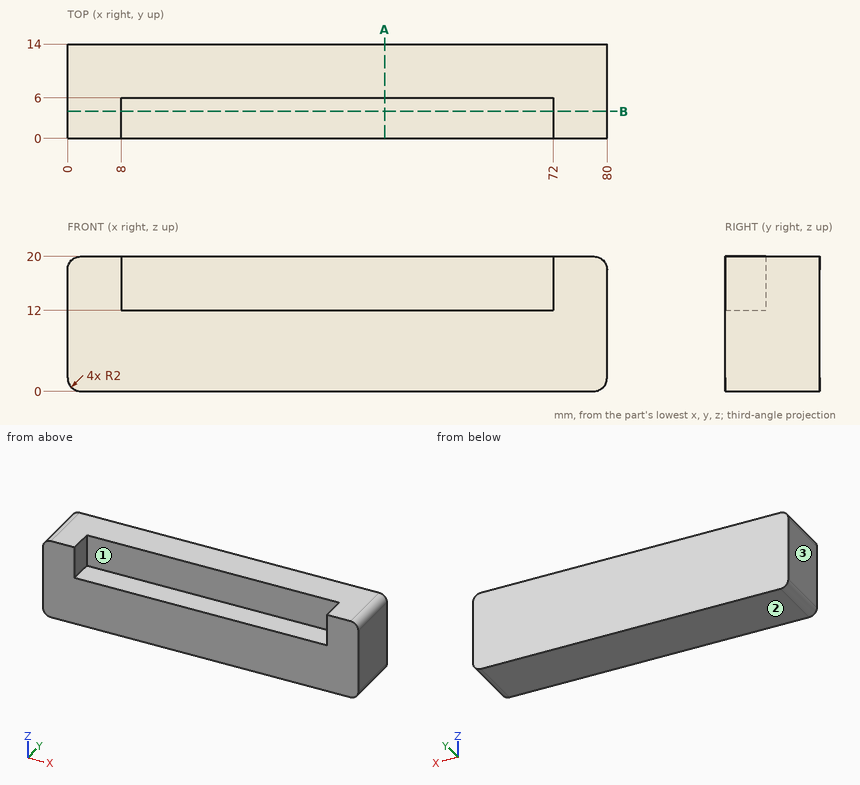
Part print with two shaded views. Sizes in mm from the minimum x, y, z corner. Round coordinates to 2 decimals unless told otherwise and drop trailing zeros. Loops run counter-clockwise (first coordinate to the right, second up) from the corner with the lowest first, then second, coordinate; pieces in that order, holes last.
Item 1: Drill centre lines: line 1 along X through (y, z) = (2.25, 16.5); line 2 along Y through (x, z) = (26, 18.5); line 3 along Z through (x, y) = (63, 5). Where is each one in solid material? Low to high.
Item 2: Saw through at A-A (x = 47). List the corners of the cut face in (y, z).
Item 3: Saw through at B-B (y = 4). List the corners of the cut face in (x, z).
Item 4: Pin check, flat tips, straight feed: P1, Ø1.5, axis at x = 12.5, y = 1.5, coming from the -Z side; P2, Ø5, axis at x = 31.5, y = 3, coming from the +Z side. Stop position of each tip, or through.
Item 5: Two-plate mould, pull along X, no slides. Class the marked faces 1, 2 and 3: released by +X, released by -X, zero draft, split by the parting line, or undercut.
Worked answers:
1. line 1: x = 0 to 8, 72 to 80
1. line 2: y = 6 to 14
1. line 3: z = 0 to 12
2. outline: (0, 0) - (14, 0) - (14, 20) - (6, 20) - (6, 12) - (0, 12) - close
3. outline: (0, 2) arc R2 ccw to (2, 0) - (78, 0) arc R2 ccw to (80, 2) - (80, 18) arc R2 ccw to (78, 20) - (72, 20) - (72, 12) - (8, 12) - (8, 20) - (2, 20) arc R2 ccw to (0, 18) - close
4. P1: stops at z = 0
4. P2: stops at z = 12
5. face 1: undercut
5. face 2: zero draft
5. face 3: released by -X
